Here's the drawing with two shaded views (mm, measured from the low corner). I have some questions. Give positions to 0.01 mm unless a question says otherwise; leave off trailing zeros. Write each loop counter-clockwise with the first axis right and the second up, starting at its lowest first coordinate (ties: lowest second). Pieces come first, ordered by that corner, then holes. Notation, with made-up numbers: M -30.75,-39 L -5.75,-39 A18 cw -5.75,-10 Z; hole C -4.75,-25.75 d1. An arc over 180 degrees is marked long. Answer as a JSON object with one key per item and string values. Group by question number.
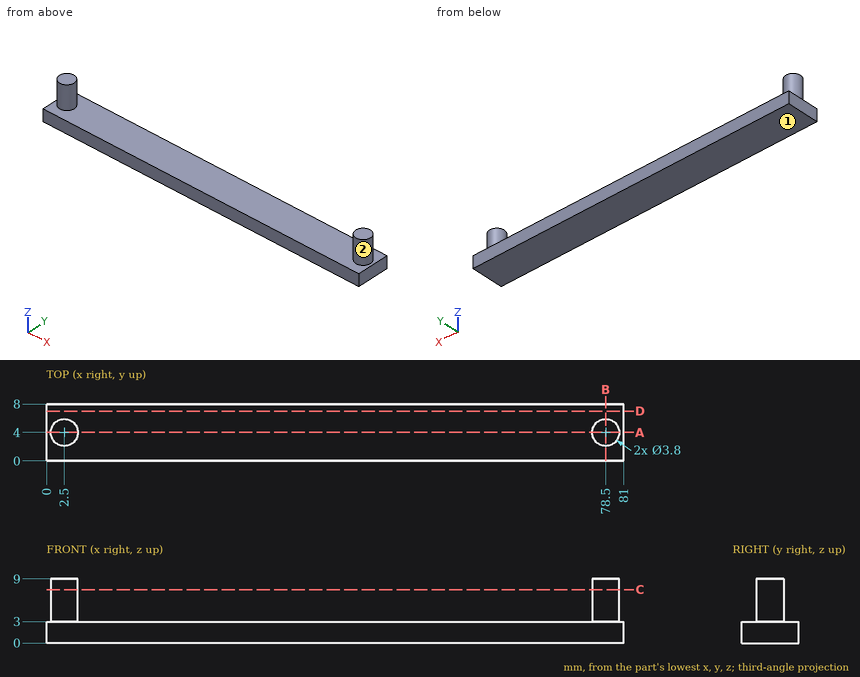
1) I'm going to push flat-ended pins straight in: pin 1 (1.5 mm diameter, centred on x = 50, z = 4, fed in from +Y); pin 2 (1 mm diameter, centred on x = 30, y = 3.5, fed in from +Z); pin 3 (4 mm diameter, centred on y = 4, z = 6, fed in from -X); pin 4 (1 mm diameter, centred on y = 3, z = 7, fed in from +X). Where does each tip first touch, or does it pass through?
2) We'd pull the mould along X, two halves only. Please class the marked faces 1 and 2: released by +X, released by -X, zero draft, split by the parting line, or undercut.
3) If we section it at B-B, the plane x = 78.5: List the corners of the cut face in (y, z) for me, plus the area to 3 significant figures.
4) Please list where these lines run through material, in increasing order: line 1 along Z through (x, y) = (55.5, 2.25); line 2 along X through (y, z) = (5.25, 7.5); line 3 along X through (y, z) = (3.75, 6). Write a range as from..to.
5) If we section it at C-C, the plane z = 7.5: List the corners of the cut face in (x, y) for me.
6) If we section it at D-D, the plane y = 7: List the corners of the cut face in (x, z) for me.
7) If we section it at A-A, the plane y = 4: List the corners of the cut face in (x, z) for me, plus the area to 3 significant figures.
Taken from the geometry:
{
 "1": {"pin 1": "through", "pin 2": "z = 3", "pin 3": "x = 0.6", "pin 4": "x = 80.33"},
 "2": {"face 1": "zero draft", "face 2": "undercut"},
 "3": {"outline": "M 0,0 L 8,0 L 8,3 L 5.9,3 L 5.9,9 L 2.1,9 L 2.1,3 L 0,3 Z", "area": "46.8 mm²"},
 "4": {"line 1": "0..3", "line 2": "1.07..3.93, 77.07..79.93", "line 3": "0.62..4.38, 76.62..80.38"},
 "5": {"outline": "C 2.5,4 d3.8; C 78.5,4 d3.8"},
 "6": {"outline": "M 0,0 L 81,0 L 81,3 L 0,3 Z"},
 "7": {"outline": "M 0,0 L 81,0 L 81,3 L 80.4,3 L 80.4,9 L 76.6,9 L 76.6,3 L 4.4,3 L 4.4,9 L 0.6,9 L 0.6,3 L 0,3 Z", "area": "289 mm²"}
}
